from build123d import *

# Parameters (mm, degrees)
F1_DEPTH = 12.7
F2_R     = 5.8193233161
F3_DEPTH = 1800


# Not quite as in the source:
# - a feature names something its author has since deleted; it is built from what else it names


with BuildPart() as f1:
    # F0 (on Front) → F1 (new body, symmetric)
    with BuildSketch(Plane.XZ):
        with BuildLine():
            Line((492.5543735346, 210), (0, 210))
            Line((0, 210), (-492.5543735346, 210))
            Line((-492.5543735346, 210), (-550, 170))
            Line((-550, 170), (-630, 170))
            Line((-630, 170), (-668.1, 170))
            Line((-668.1, 170), (-668.1, -230))
            Line((-668.1, -230), (-668.1, -330))
            Line((-668.1, -330), (-630, -330))
            Line((-630, -330), (-630, -280))
            Line((-630, -280), (-600, -280))
            Line((-600, -280), (-600, -330))
            Line((-600, -330), (-580, -330))
            Line((-580, -330), (-580, -236.35))
            ThreePointArc((-580, -236.35), (-581.8598719395, -231.8598719395), (-586.35, -230))
            Line((-586.35, -230), (-630, -230))
            Line((-630, -230), (-630, -50))
            Line((-630, -50), (630, 0))
            Line((630, 0), (630, -50))
            Line((630, -50), (630, -230))
            Line((630, -230), (586.35, -230))
            ThreePointArc((586.35, -230), (581.8598719395, -231.8598719395), (580, -236.35))
            Line((580, -236.35), (580, -330))
            Line((580, -330), (600, -330))
            Line((600, -330), (600, -280))
            Line((600, -280), (630, -280))
            Line((630, -280), (630, -330))
            Line((630, -330), (668.1, -330))
            Line((668.1, -330), (668.1, -230))
            Line((668.1, -230), (668.1, 170))
            Line((668.1, 170), (630, 170))
            Line((630, 170), (550, 170))
            Line((550, 170), (492.5543735346, 210))
        make_face()
        Polygon((550, 43.6507936508), (-550, 0), (-550, 128.1044334173), (-492.5543735346, 168.1044334173), (492.5543735346, 168.1044334173), (550, 128.1044334173), align=None, mode=Mode.SUBTRACT)
    extrude(amount=F1_DEPTH, both=True)

    # F2 (on face) → F3 (cut)
    with BuildSketch(Plane.YZ.offset(668.1)):
        with Locations((0, -307.489156723)):
            Circle(F2_R)
    extrude(amount=-F3_DEPTH, mode=Mode.SUBTRACT)


solid = f1.part
Input: part model. Units: mm. Frame: model coordinates. A direction names the side the tool comes from. Coordinates: 2 decimals unless noted, no trailing zeros. Loops run counter-clockwise (first coordinate to the right, second up) from the corner with the lowest first, then second, coordinate; pieces in that order, holes last.
Q1. Cut plane A-A (z = 64). Output: boundary loops of the cut face in (x, y), then the cut area to 3 significant figures.
Q2. Cut plane B-B (x = -210). Output: boundary loops of the cut face in (y, z).
Q3. Material intervals for line 1 (X direction, y = -5, z = -251.5); line 2 (X direction, y = -8, z = 77.5); line 3 (Z direction, x = -654, y = 0), sorted ascending.
Q4. Contact query for flat-ended pins moving along their axis: pin 1 (6 mm diameter, centred on x = -61, y = 0, fed in from -Z); pin 2 (7.5 mm diameter, centred on x = -605.5, y = -4, fed in from +Z); pin 3 (12.5 mm diameter, centred on y = 4.5, z = -308.5, fed in from +X); pin 4 (10 mm diameter, centred on x = 393.5, y = 7, fed in from -Z). Output: stop coordinate, or through.
Q5. Cut plane C-C (y = 0). Give the number of separate pieces and of enclosed holes in the cut face, then the cut area to 3 significant figures.
Q6. Set-up query: faces 4 (the face through (7, 0, 210)), 5 (the face through (610, 0, 170)), 6 (the face through (-550, 0, 63)), 7 (the face through (615, 0, -280)). Return all of +Z, -Z, +X, -X, +Y, -Y with unobstructed straight access to the full face (end or side cutting, diameter ignored); none if empty.
Q7. Draft query along X for faces 1 (the face through (649, 0, -330)), 2 (the face through (-668.1, 0, -77)), 3 (the face through (-7, 0, 168.104)). Return one class per face: +X half, -X half, draft (parallel to the pull), parting line (faces both ways), or undercut.
Working result:
1. outline: (-668.1, -12.7) - (-550, -12.7) - (-550, 12.7) - (-668.1, 12.7) - close; (550, -12.7) - (668.1, -12.7) - (668.1, 12.7) - (550, 12.7) - close
1. area: 6,000 mm2
2. outline: (-12.7, -33.33) - (12.7, -33.33) - (12.7, 13.49) - (-12.7, 13.49) - close; (-12.7, 168.1) - (12.7, 168.1) - (12.7, 210) - (-12.7, 210) - close
3. line 1: x = -668.1 to -580, 580 to 668.1
3. line 2: x = -668.1 to -550, 550 to 668.1
3. line 3: z = -330 to -313.31, -301.67 to 170
4. pin 1: stops at z = -27.54
4. pin 2: stops at z = 170
4. pin 3: stops at x = 668.1
4. pin 4: stops at z = -9.58
5. separate pieces: 5
5. enclosed holes: 1
5. area: 173,000 mm2
6. face 4: +Z, +X, -X, +Y, -Y
6. face 5: +Z, +X, +Y, -Y
6. face 6: +Y, -Y
6. face 7: -Z, +Y, -Y
7. face 1: draft
7. face 2: -X half
7. face 3: undercut
